Geometry check sheet. Reference: drawing and pictorial views, mm from the part's lowest x, y, z. A direction names the side the tool comes from. Give positions to 0.01 mm unless a question says otherwise; leave off trailing zeros. Order: outer loops, then holes, each group sorted by start corner. A loop starts at its lowest first (then second) coordinate and runs counter-clockwise, first axis right, second up.
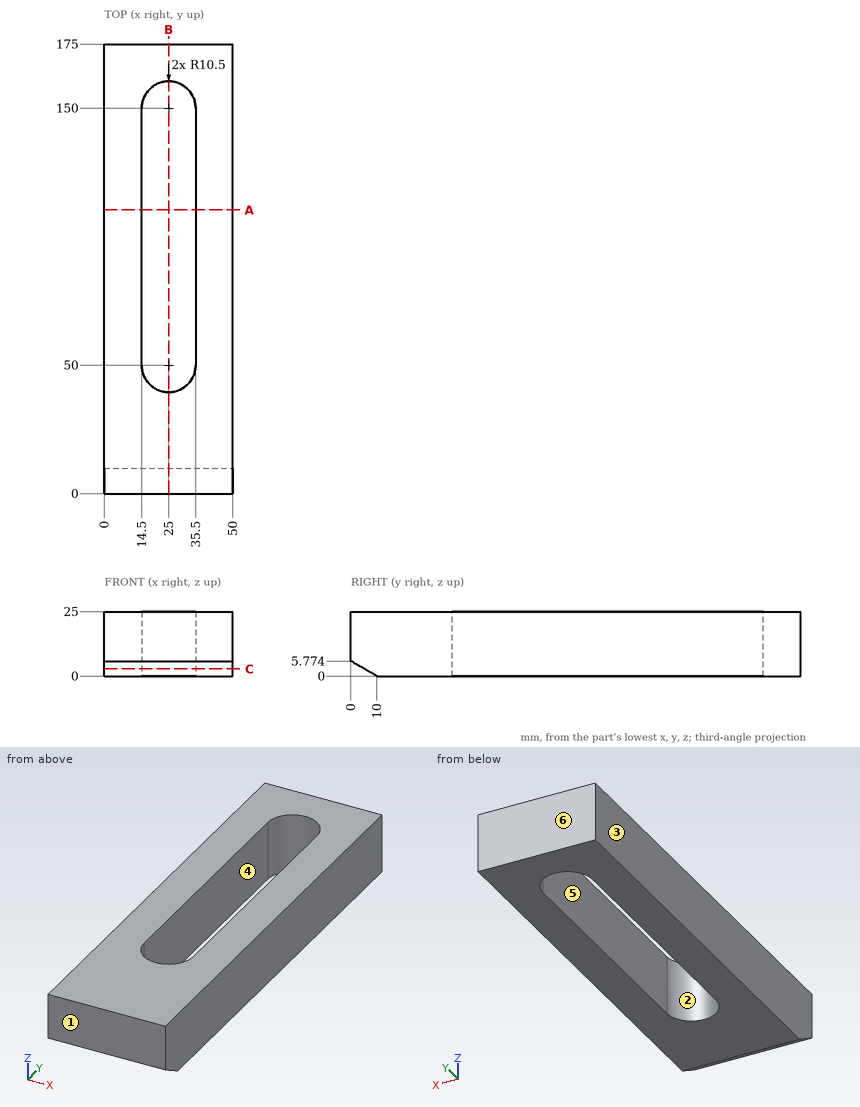
(1) Release check for a two-part mould opening along X. For the marked faces 3, 4, 5 and 6 record: released by +X, released by -X, zero draft, split by the parting line, or undercut.
Response values:
face 3: released by -X
face 4: undercut
face 5: undercut
face 6: zero draft
(2) Gauge pin test, flat end, axial feed: pin 1 Ø8 at (x, y) = (15.5, 29) entering from -Z. Record the tip position at first contact, or that the pin passes through.
Response values:
pin 1: stops at z = 0
(3) Cross-section at B-B on x = 25. Enter the section's corners in (y, z), then the cut area to 3 significant figures.
Response values:
outline: (0, 5.77) - (10, 0) - (39.5, 0) - (39.5, 25) - (0, 25) - close; (160.5, 0) - (175, 0) - (175, 25) - (160.5, 25) - close
area: 1,320 mm2
(4) Material ranges on L1, parallel to X at y = 119.5, z = 5.5; L2, parallel to Y at x = 23, z = 14; L3, parallel to X at y = 153.5, z = 1, recorded low to high.
Response values:
L1: x = 0 to 14.5, 35.5 to 50
L2: y = 0 to 39.69, 160.31 to 175
L3: x = 0 to 15.1, 34.9 to 50
(5) Cross-section at C-C on z = 2.75. Enter the section's corners in (x, y).
Response values:
outline: (0, 5.24) - (50, 5.24) - (50, 175) - (0, 175) - close; hole (14.5, 50) arc R10.5 ccw to (35.5, 50) - (35.5, 150) arc R10.5 ccw to (14.5, 150) - close
(6) Cross-section at A-A on y = 110.5. Enter the section's corners in (x, z), then the cut area to 3 significant figures.
Response values:
outline: (0, 0) - (14.5, 0) - (14.5, 25) - (0, 25) - close; (35.5, 0) - (50, 0) - (50, 25) - (35.5, 25) - close
area: 725 mm2
(7) Set-up check for the marked faces 1 and 2: record each of +Z, -Z, +X, -X, +Y, -Y from which the full face is reachable in a straight line by a thin tool's end or side.
Response values:
face 1: +Z, -Z, +X, -X, -Y
face 2: +Z, -Z
